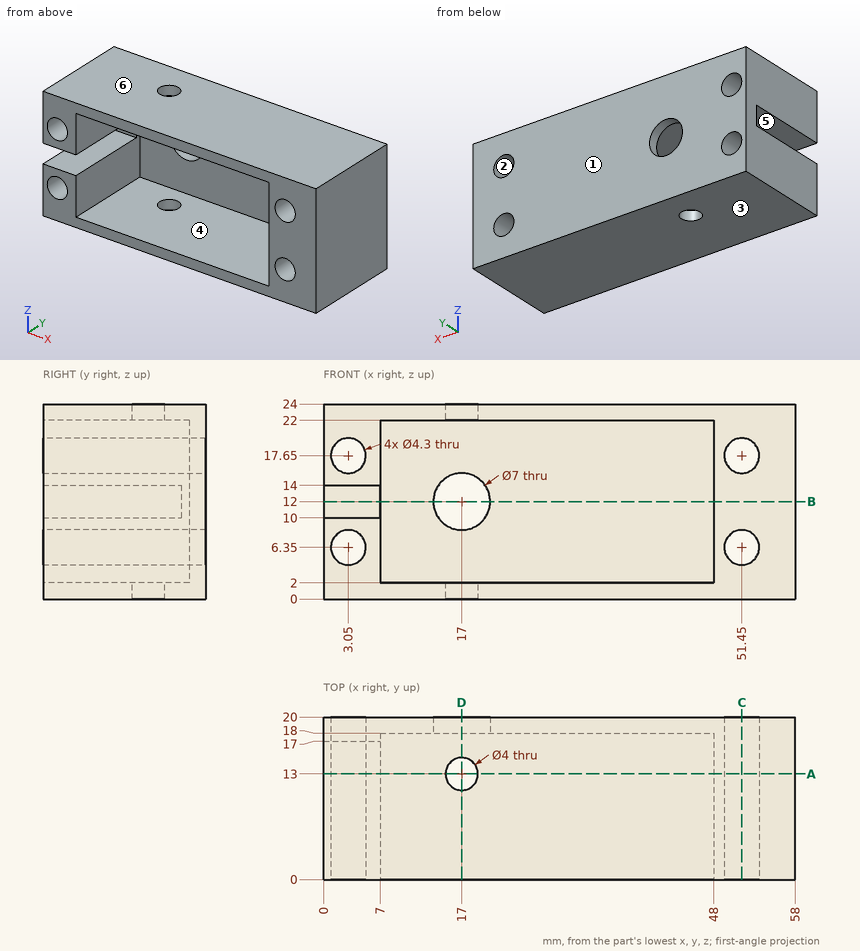
Study the drawing (mm; zero at the part's minimum x, y, z) and answer. A direction names the side the tool comes from. Give positions to 0.01 mm unless a question says otherwise; leave off trailing zeros. Write each loop counter-clockwise with the first axis right and the second up, starting at its lowest first coordinate (ties: lowest second). Pieces come first, ordered by that corner, then holes. Notation, with made-up numbers: (34, 73.25) - (93, 73.25) arc R14 ccw to (93, 84.25) - close; hole circle Ø10 at (34.25, 80.5). An arc over 180 degrees is marked (long way). Write item = value, one per line. Start each with the question number.
Item 1: Find section C-C (x = 51.45). Give the vertices of the cut face in (y, z), then the cut area to 3 significant figures.
Item 2: Each of these flat-tipped pins is pushed along its axis until it touches: P1, Ø1.2, axis at x = 5, z = 12, coming from the -Y side; P2, Ø10, axis at x = 32.5, z = 16.5, coming from the -Y side. Where does it stop, or does it pass through?
Item 3: A tool of negligible diameter and unlimited length cuts with its end or side. For the marked faces 4, 5 and 6, from which of +Z, -Z, +X, -X, +Y, -Y can it reach the whole face along a straight path? Write none if from no direction.
Item 4: Find section D-D (x = 17). Give the vertices of the cut face in (y, z).
Item 5: Find section A-A (y = 13). Give the vertices of the cut face in (x, z).
Item 6: Find the intervals of material crossed by probe 1 along X at (y, z) = (6, 6.35); probe 2 along X at (y, z) = (8.5, 14.5); probe 3 along Z at (x, y) = (30.5, 9.75), in increasing order. Write a range as [from, to].
Item 7: Find section B-B (z = 12). Give the vertices of the cut face in (x, y), then the cut area to 3 significant figures.
Item 8: The mould has two halves that part along Z. Classify the marked faces 1, 2 and 3: +Z half, -Z half, draft (parallel to the pull), parting line (faces both ways), or undercut.
Response:
q1.outline = (0, 0) - (20, 0) - (20, 4.2) - (0, 4.2) - close; (0, 8.5) - (20, 8.5) - (20, 15.5) - (0, 15.5) - close; (0, 19.8) - (20, 19.8) - (20, 24) - (0, 24) - close
q1.area = 308 mm²
q2.P1 = 17
q2.P2 = 18
q3.face_4 = -Y
q3.face_5 = -X, -Y
q3.face_6 = +Z, +X, -X, +Y, -Y
q4.outline = (0, 0) - (11, 0) - (11, 2) - (0, 2) - close; (0, 22) - (11, 22) - (11, 24) - (0, 24) - close; (15, 0) - (20, 0) - (20, 8.5) - (18, 8.5) - (18, 2) - (15, 2) - close; (15, 22) - (18, 22) - (18, 15.5) - (20, 15.5) - (20, 24) - (15, 24) - close
q5.outline = (0, 0) - (15, 0) - (15, 2) - (7, 2) - (7, 10) - (0, 10) - close; (0, 14) - (7, 14) - (7, 22) - (15, 22) - (15, 24) - (0, 24) - close; (19, 0) - (58, 0) - (58, 24) - (19, 24) - (19, 22) - (48, 22) - (48, 2) - (19, 2) - close; hole circle Ø4.3 at (3.05, 6.35); hole circle Ø4.3 at (3.05, 17.65); hole circle Ø4.3 at (51.45, 6.35); hole circle Ø4.3 at (51.45, 17.65)
q6.probe_1 = [0, 0.9], [5.2, 7], [48, 49.3], [53.6, 58]
q6.probe_2 = [0, 7], [48, 58]
q6.probe_3 = [0, 2], [22, 24]
q7.outline = (0, 17) - (7, 17) - (7, 18) - (13.5, 18) - (13.5, 20) - (0, 20) - close; (20.5, 18) - (48, 18) - (48, 0) - (58, 0) - (58, 20) - (20.5, 20) - close
q7.area = 289 mm²
q8.face_1 = draft
q8.face_2 = undercut
q8.face_3 = -Z half
